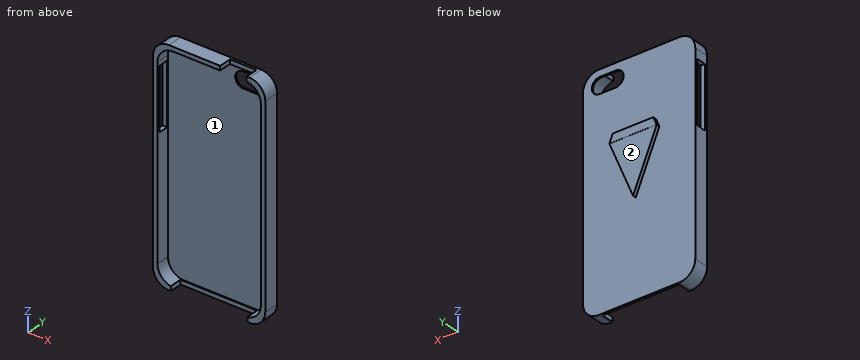
```python
from build123d import *

# Parameters (mm, degrees)
F1_DEPTH  = 8.6
F3_DEPTH  = 7.7
F5_DEPTH  = 5
F7_DEPTH  = 1
F8_W      = 43.4
F8_H      = 7.1749998596
F9_DEPTH  = 25
F10_W     = 15
F10_H     = 7.1
F11_DEPTH = 25
F12_W     = 5.6
F12_H     = 35
F13_DEPTH = 25
F15_DEPTH = 1
F17_DEPTH = 0.95


# Not quite as in the source:
# - a feature names something its author has since deleted; it is built from what else it names


with BuildPart() as f1:
    # F0 (on Front) → F1 (new body)
    with BuildSketch(Plane.XZ):
        with BuildLine():
            Line((34.2577553943, 74.9795119995), (-11.3422446057, 74.9795119995))
            ThreePointArc((-11.3422446057, 74.9795119995), (-17.7062056364, 72.3434730302), (-20.3422446057, 65.9795119995))
            Line((-20.3422446057, 65.9795119995), (-20.3422446057, -44.8204880005))
            ThreePointArc((-20.3422446057, -44.8204880005), (-17.7062056364, -51.1844490312), (-11.3422446057, -53.8204880005))
            Line((-11.3422446057, -53.8204880005), (34.2577553943, -53.8204880005))
            ThreePointArc((34.2577553943, -53.8204880005), (40.621716425, -51.1844490312), (43.2577553943, -44.8204880005))
            Line((43.2577553943, -44.8204880005), (43.2577553943, 65.9795119995))
            ThreePointArc((43.2577553943, 65.9795119995), (40.621716425, 72.3434730302), (34.2577553943, 74.9795119995))
        make_face()
    extrude(amount=F1_DEPTH)

    # F2 (on face) → F3 (cut)
    with BuildSketch(Plane.XZ.offset(8.6)):
        with BuildLine():
            Line((31.7577553943, 72.4795119995), (-8.8422446057, 72.4795119995))
            ThreePointArc((-8.8422446057, 72.4795119995), (-15.2062056364, 69.8434730302), (-17.8422446057, 63.4795119995))
            Line((-17.8422446057, 63.4795119995), (-17.8422446057, -42.3204880005))
            ThreePointArc((-17.8422446057, -42.3204880005), (-15.2062056364, -48.6844490312), (-8.8422446057, -51.3204880005))
            Line((-8.8422446057, -51.3204880005), (31.7577553943, -51.3204880005))
            ThreePointArc((31.7577553943, -51.3204880005), (38.121716425, -48.6844490312), (40.7577553943, -42.3204880005))
            Line((40.7577553943, -42.3204880005), (40.7577553943, 63.4795119995))
            ThreePointArc((40.7577553943, 63.4795119995), (38.121716425, 69.8434730302), (31.7577553943, 72.4795119995))
        make_face()
    extrude(amount=-F3_DEPTH, mode=Mode.SUBTRACT)

    # F4 (on face) → F5 (cut)
    with BuildSketch(Plane(origin=(0, 0, 0), x_dir=(-1, 0, 0), z_dir=(0, 1, 0))):
        with BuildLine():
            Line((-24.7577553943, 70.9795119995), (-33.7577553943, 70.9795119995))
            ThreePointArc((-33.7577553943, 70.9795119995), (-36.9397359096, 69.6614925148), (-38.2577553943, 66.4795119995))
            ThreePointArc((-38.2577553943, 66.4795119995), (-36.9397359096, 63.2975314842), (-33.7577553943, 61.9795119995))
            Line((-33.7577553943, 61.9795119995), (-24.7577553943, 61.9795119995))
            ThreePointArc((-24.7577553943, 61.9795119995), (-21.5757748789, 63.2975314842), (-20.2577553943, 66.4795119995))
            ThreePointArc((-20.2577553943, 66.4795119995), (-21.5757748789, 69.6614925148), (-24.7577553943, 70.9795119995))
        make_face()
    extrude(amount=-F5_DEPTH, mode=Mode.SUBTRACT)

    # F6 (on face) → F7 (join)
    with BuildSketch(Plane(origin=(0, 0, 0), x_dir=(-1, 0, 0), z_dir=(0, 1, 0))):
        Polygon((-24.8744231037, 36.9551813005), (-26.7878402656, 32.3357836379), (-13.3939201328, 0), (0, 32.3357836379), (-1.9134171618, 36.9551813005), align=None)
    extrude(amount=F7_DEPTH)

    # F8 (on face) → F9 (cut)
    with BuildSketch(Plane(origin=(0, 0, -53.8204880005), x_dir=(1, 0, 0), z_dir=(0, 0, -1))):
        with Locations((11.4577553943, 5.0125000702)):
            Rectangle(F8_W, F8_H)
    extrude(amount=-F9_DEPTH, mode=Mode.SUBTRACT)

    # F10 (on face) → F11 (cut)
    with BuildSketch(Plane.XY.offset(74.9795119995)):
        with Locations((25.2577553943, -5.05)):
            Rectangle(F10_W, F10_H)
    extrude(amount=-F11_DEPTH, mode=Mode.SUBTRACT)

    # F12 (on face) → F13 (cut)
    with BuildSketch(Plane(origin=(-20.3422446057, 0, 0), x_dir=(0, -1, 0), z_dir=(-1, 0, 0))):
        with Locations((4.3, 43.4795119995)):
            Rectangle(F12_W, F12_H)
    extrude(amount=-F13_DEPTH, mode=Mode.SUBTRACT)

    # F14 (on face) → F15 (join)
    with BuildSketch(Plane(origin=(0, 1, 0), x_dir=(-1, 0, 0), z_dir=(0, 1, 0))):
        Polygon((-24.8744231037, 36.9551813005), (-26.7878402656, 32.3357836379), (0, 32.3357836379), (-1.9134171618, 36.9551813005), align=None)
    extrude(amount=F15_DEPTH)

    # F16 (on face) → F17 (join)
    with BuildSketch(Plane(origin=(0, 1, 0), x_dir=(-1, 0, 0), z_dir=(0, 1, 0))):
        Polygon((0, 32.3357836379), (-26.7878402656, 32.3357836379), (-13.3939201328, 0), align=None)
    extrude(amount=F17_DEPTH)


solid = f1.part
```
CAD build for the part. Positions are in the model's coordinates, mm. Face numbers are marked on the shaded views. Round coordinates to 2 decimals unless told otherwise and drop trailing zeros. Loops run counter-clockwise (first coordinate to the right, second up) from the corner with the lowest first, then second, coordinate; pieces in that order, holes last. Notation, with made-up numbers: M 88,64 L 110,64 A20 ccw 110,82 Z; hole C 66,-26.75 d8. An arc over 180 degrees is marked long. Return JSON: item names as keys, results as strings. Group by question number.
(1) Mould opens along Z. For the marked faces 1 and 2 say: +Z half, -Z half, draft (parallel to the pull), parting line (faces both ways), or undercut.
(2) Saw through at A-A, the plane z = 58. List the corners of the cut face in (x, y).
(3) Saw through at D-D, the plane x = 22. List the corners of the cut face in (y, z) (3 decimals).
(4) Drop flat-ended pins along their axis: P1, Ø0.8, axis at x = -18.5, z = 48, coming from the +Y side; P2, Ø2, axis at x = 18, y = 1.5, coming from the +Z side; P3, Ø0.8, axis at x = -19.5, y = -3, coming from the -Z side. Give the stop position or say it passes through.
(5) Saw through at B-B, the plane y = -3.75. List the corners of the cut face in (x, z), and give its area (3 significant figures).
(6) Saw through at C-C, the plane z = -20.5. List the corners of the cut face in (x, y).
(7) Wall check: probe 1 along X at (y, z) = (-7.25, 45.5); probe 2 along Y at (x, z) = (-6.5, -33.5); probe 3 along Z at (x, y) = (7.5, -5.25). Give the ranges that are in metal, low to high. Write a range as [from, to].
Answer list:
{
 "1": {"face 1": "undercut", "face 2": "draft"},
 "2": {"outline": "M -20.34,-8.6 L -17.84,-8.6 L -17.84,-7.1 L -20.34,-7.1 Z; M -20.34,-1.5 L -17.84,-1.5 L -17.84,-0.9 L 40.76,-0.9 L 40.76,-8.6 L 43.26,-8.6 L 43.26,0 L -20.34,0 Z"},
 "3": {"outline": "M -1.5,72.48 L -0.9,72.48 L -0.9,70.035 L 0,70.035 L 0,74.98 L -1.5,74.98 Z; M -1.425,-53.82 L 0,-53.82 L 0,20.777 L 1.95,20.777 L 1.95,32.336 L 2,32.336 L 2,36.955 L 0,36.955 L 0,62.924 L -0.9,62.924 L -0.9,-51.32 L -1.425,-51.32 Z"},
 "4": {"P1": "y = 0", "P2": "z = 36.96", "P3": "z = -49.38"},
 "5": {"outline": "M -20.34,-44.82 A9 ccw -11.34,-53.82 L -10.24,-53.82 L -10.24,-51.21 A9 cw -17.84,-42.32 L -17.84,25.98 L -20.34,25.98 Z; M -20.34,60.98 L -17.84,60.98 L -17.84,63.48 A9 cw -8.84,72.48 L 17.76,72.48 L 17.76,74.98 L -11.34,74.98 A9 ccw -20.34,65.98 Z; M 32.76,72.42 A9 cw 40.76,63.48 L 40.76,-42.32 A9 cw 33.16,-51.21 L 33.16,-53.82 L 34.26,-53.82 A9 ccw 43.26,-44.82 L 43.26,65.98 A9 ccw 34.26,74.98 L 32.76,74.98 Z", "area": "703 mm2"},
 "6": {"outline": "M -20.34,-8.6 L -17.84,-8.6 L -17.84,-0.9 L 40.76,-0.9 L 40.76,-8.6 L 43.26,-8.6 L 43.26,0 L -20.34,0 Z"},
 "7": {"probe 1": "[-20.34, -17.84], [40.76, 43.26]", "probe 2": "[-0.9, 0]", "probe 3": "[72.48, 74.98]"}
}
